Study the drawing (mm; zero at the part's minimum x, y, z) and answer. Give positions to 0.01 mm unless a question says otherwise; leave off trailing zeros. Order: outer loops, then holes, each group sorted by start corner. A loop starts at its lowest first (then second) coordinate and runs counter-clockwise, first axis right, second up. Notation, with made-up numbers: (-38.75, 73) -> (19.25, 73) arc R14 ccw to (19.25, 90) -> close; hole circle Ø10 at (47.5, 79). An arc over 180 degrees is marked (long way). One line per question, with ' | ' between items. Start each with the question number.
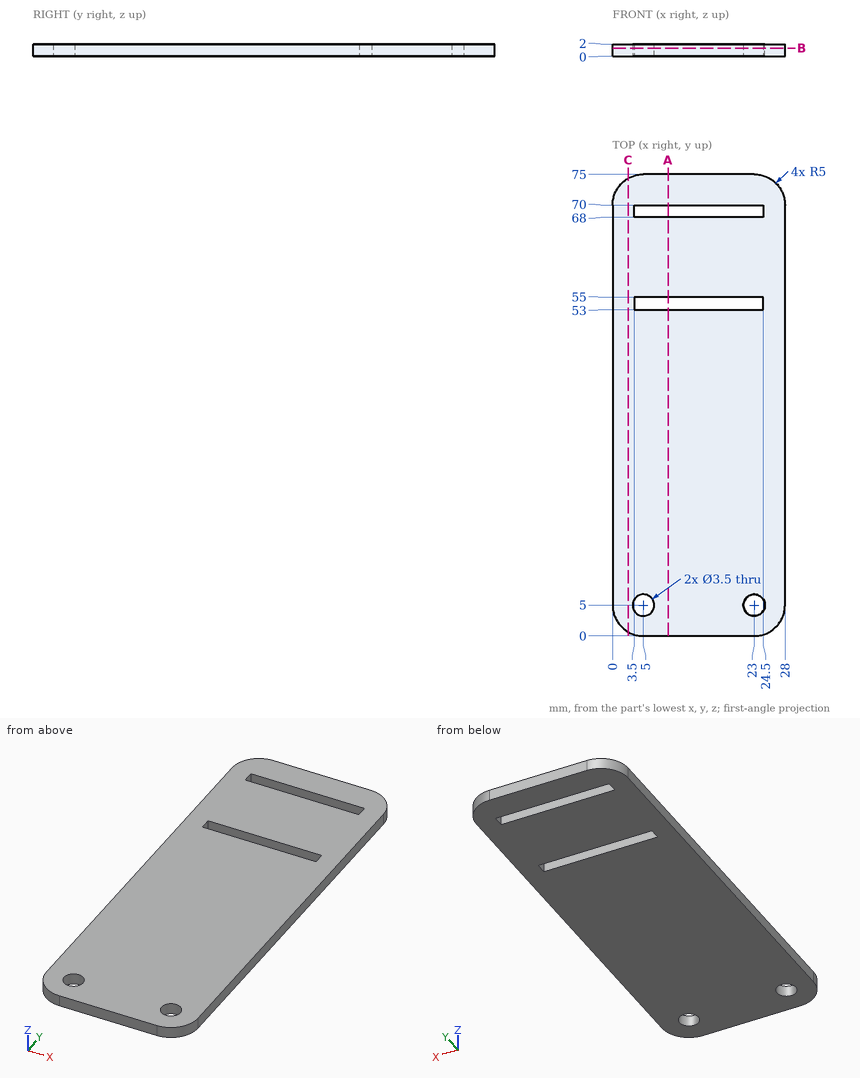
Q1. A cutting plane is placed at B-B, the plane z = 1.35. Determine the outline of the cut face in (x, y).
Q2. A cutting plane is placed at A-A, the plane x = 9. Determine the outline of the cut face in (y, z), then the cut area to 3 significant figures.
Q3. Find the intervals of material crossed by line 1 (Y direction, x = 8.25, z = 0.4); line 2 (Y direction, x = 5, z = 0.5); line 3 (Y direction, x = 6, z = 0.2), in increasing order.
Q4. Given P1, Ø3, axis at x = 23, y = 5, coming from the -Z side, flat-ended and moving along its own axis, determine where the tip first touches the part or whether it passes through.
Q5. A cutting plane is placed at C-C, the plane x = 2.5. Determine the outline of the cut face in (y, z), then the cut area to 3 significant figures.
Geometry results:
1) outline: (0, 5) arc R5 ccw to (5, 0) -> (23, 0) arc R5 ccw to (28, 5) -> (28, 70) arc R5 ccw to (23, 75) -> (5, 75) arc R5 ccw to (0, 70) -> close; hole circle Ø3.5 at (5, 5); hole (3.5, 53) -> (24.5, 53) -> (24.5, 55) -> (3.5, 55) -> close; hole (3.5, 68) -> (24.5, 68) -> (24.5, 70) -> (3.5, 70) -> close; hole circle Ø3.5 at (23, 5)
2) outline: (0, 0) -> (53, 0) -> (53, 2) -> (0, 2) -> close; (55, 0) -> (68, 0) -> (68, 2) -> (55, 2) -> close; (70, 0) -> (75, 0) -> (75, 2) -> (70, 2) -> close | area: 142 mm²
3) line 1: 0 to 53, 55 to 68, 70 to 75 | line 2: 0 to 3.25, 6.75 to 53, 55 to 68, 70 to 75 | line 3: 0 to 3.56, 6.44 to 53, 55 to 68, 70 to 75
4) P1: through
5) outline: (0.67, 0) -> (74.33, 0) -> (74.33, 2) -> (0.67, 2) -> close | area: 147 mm²
